Part model, mm, in its own coordinate system. Face numbers are marked on the shaded views. Round coordinates to 2 decimals unless told otherwise and drop trailing zeros. Write each loop counter-clockwise with the first axis right and the second up, starting at its lowest first coordinate (ties: lowest second). Pieces come first, ordered by that corner, then holes. Notation, with made-up numbers: (-3, 40.25) -> (47, 40.25) arc R10 cw to (47, 50.25) -> close; hole circle Ø6 at (64.5, -2.5). An arc over 180 degrees is marked (long way). Use CSV: the item, a comma, the result in double quotes. Start each with the question number.
(1) Two-plate mould, pull along X, no slides. Class the marked faces 1 and 2: released by +X, released by -X, zero draft, split by the parting line, or undercut.
(2) Drop flat-ended pins along their axis: pin 1 (1.3 mm diameter, centred on y = 21.5, z = 2, fed in from -X); pin 2 (1 mm diameter, centred on x = 11.5, y = 14.5, fed in from -Z); pin 3 (2 mm diameter, centred on y = 7, z = 4, fed in from +X); pin 4 (2 mm diameter, centred on x = 8.5, y = 6, fed in from -Z). Give the stop position or say it passes through.
(3) Saw through at A-A (y = 0). Give the cut face in (x, z), plus the area to 3 significant figures.
(4) Saw through at B-B (y = 21.5). Give the cut face in (x, z), plus the area to 3 significant figures.
(5) Probe line 1 (Y direction, x = 0, z = 1.45); line 2 (Y direction, x = -15, z = 3.6); line 3 (Z direction, x = -17, y = 6). List the from-to ranges inside material, lowest first. Write a range as [from, to].
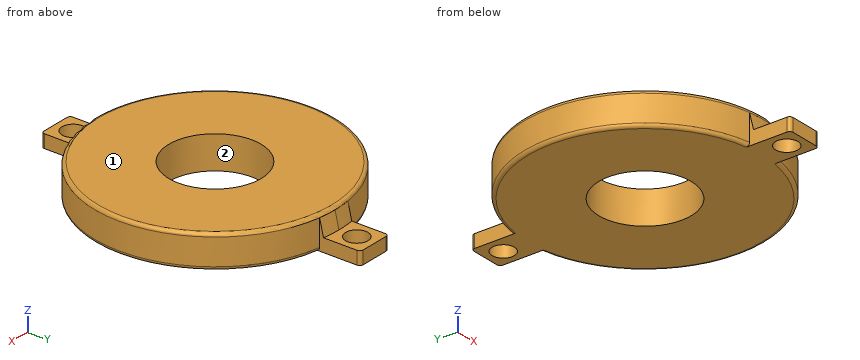
```python
from build123d import *
from OCP.BRepFilletAPI import BRepFilletAPI_MakeChamfer

# Parameters (mm, degrees)
CROQUIS2_R              = 18.2
CROQUIS2_R_2            = 7
SALIENTE_EXTRUIR1_DEPTH = 5
CROQUIS2_3_R            = 1.7
SALIENTE_EXTRUIR2_DEPTH = 2
REDONDEO1_R             = 0.5
REDONDEO4_R             = 0.5
CHAFL_N2_SIZE           = 0.6
CHAFL_N2_SIZE_2         = 2.5


with BuildPart() as part:
    # Croquis2 → Saliente-Extruir1 (new body)
    with BuildSketch(Plane(origin=(0, 0, 0), x_dir=(0, 1, 0), z_dir=(0, 0, 1))):
        with Locations(Location((0, 0, 0), (0, 0, 270))):
            Circle(CROQUIS2_R)
        with Locations(Location((0, 0, 0), (0, 0, 270))):
            Circle(CROQUIS2_R_2, mode=Mode.SUBTRACT)
    extrude(amount=SALIENTE_EXTRUIR1_DEPTH)

    # Croquis2<3> → Saliente-Extruir2 (add)
    # profile 1 of 2: a face of its own
    with BuildSketch(Plane(origin=(0, 0, 0), x_dir=(0, 1, 0), z_dir=(0, 0, 1))):
        with BuildLine():
            Line((-24.2, -2.7), (-17.998611058, -2.7))
            ThreePointArc((-17.998611058, -2.7), (-18.2, 0), (-17.998611058, 2.7))
            Line((-17.998611058, 2.7), (-24.2, 2.7))
            Line((-24.2, 2.7), (-24.2, -2.7))
        make_face()
        with Locations(Location((-21.5, 0, 0), (0, 0, 270))):
            Circle(CROQUIS2_3_R, mode=Mode.SUBTRACT)
    # profile 2 of 2: a face of its own
    with BuildSketch(Plane(origin=(0, 0, 0), x_dir=(0, 1, 0), z_dir=(0, 0, 1))):
        with BuildLine():
            ThreePointArc((18.2, 0), (18.149582932, -1.353750116), (17.998611058, -2.7))
            Line((17.998611058, -2.7), (24.2, -2.7))
            Line((24.2, -2.7), (24.2, 2.7))
            Line((24.2, 2.7), (17.998611058, 2.7))
            ThreePointArc((17.998611058, 2.7), (18.149582932, 1.353750116), (18.2, 0))
        make_face()
        with Locations(Location((21.5, 0, 0), (0, 0, 270))):
            Circle(CROQUIS2_3_R, mode=Mode.SUBTRACT)
    extrude(amount=SALIENTE_EXTRUIR2_DEPTH)

    # Redondeo1
    redondeo1_edges = [part.edges().sort_by_distance(p)[0] for p in [
        (-2.7, -24.2, 1),
        (2.7, -24.2, 1),
        (2.7, 24.2, 1),
        (-2.7, 24.2, 1),
    ]]
    fillet(redondeo1_edges, radius=REDONDEO1_R)

    # Redondeo4
    redondeo4_edges = [part.edges().sort_by_distance(p)[0] for p in [
        (13.790939054, 11.87644728, 0),
        (-18.2, 0, 5),
        (-18.2, 0, 0),
    ]]
    fillet(redondeo4_edges, radius=REDONDEO4_R)

    # Chaflán2
    chafl_n2_edges_1 = [part.edges().sort_by_distance(p)[0] for p in [
        (0, -18.2, 2),
    ]]
    chafl_n2_side_1 = [part.faces().sort_by_distance(p)[0] for p in [
        (0, -18.212, 2),
    ]]
    chafl_n2_edges_2 = [part.edges().sort_by_distance(p)[0] for p in [
        (0, 18.2, 2),
    ]]
    chafl_n2_side_2 = [part.faces().sort_by_distance(p)[0] for p in [
        (0, 18.2, 2.012),
    ]]
    chafl_n2 = BRepFilletAPI_MakeChamfer(part.part.solid().wrapped)
    for e in chafl_n2_edges_1:
        chafl_n2.Add(CHAFL_N2_SIZE - 0.0001, CHAFL_N2_SIZE_2 - 0.0001, e.wrapped, chafl_n2_side_1[0].wrapped)
    for e in chafl_n2_edges_2:
        chafl_n2.Add(CHAFL_N2_SIZE_2 - 0.0001, CHAFL_N2_SIZE - 0.0001, e.wrapped, chafl_n2_side_2[0].wrapped)
    add(Compound.cast(chafl_n2.Shape()), mode=Mode.REPLACE)  # a hair under: the kernel refuses the full size


solid = part.part
```
Answers:
1,face 1,"zero draft"
1,face 2,"undercut"
2,pin 1,"stops at x = -2.7"
2,pin 2,"stops at z = 0.11"
2,pin 3,"stops at x = 17.18"
2,pin 4,"stops at z = 0"
3,outline,"(-18.2, 0.5) arc R0.5 ccw to (-17.7, 0) -> (-7, 0) -> (-7, 5) -> (-17.7, 5) arc R0.5 ccw to (-18.2, 4.5) -> close; (7, 0) -> (17.7, 0) arc R0.5 ccw to (18.2, 0.5) -> (18.2, 4.5) arc R0.5 ccw to (17.7, 5) -> (7, 5) -> close"
3,area,"112 mm²"
4,outline,"(-2.7, 0) -> (-1.7, 0) -> (-1.7, 2) -> (-2.7, 2) -> close; (1.7, 0) -> (2.7, 0) -> (2.7, 2) -> (1.7, 2) -> close"
4,area,"4.00 mm²"
5,line 1,"y = [-24.2, -23.2], [-19.8, -7], [7, 19.8], [23.2, 24.2]"
5,line 2,"y = [-10.31, 10.31]"
5,line 3,"z = [0.12, 4.88]"
